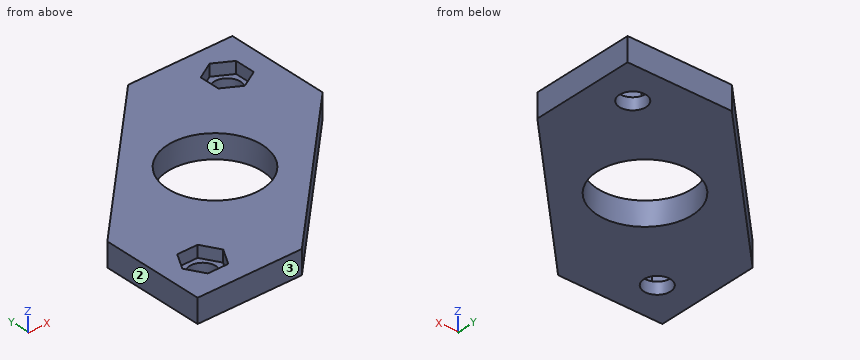
```python
from build123d import *

# Parameters (mm, degrees)
SKETCH1_R           = 8
SKETCH1_R_2         = 2.25
BOSS_EXTRUDE1_DEPTH = 4
CUT_EXTRUDE1_DEPTH  = 2


with BuildPart() as part:
    # Sketch1 → Boss-Extrude1 (new body)
    with BuildSketch(Plane.XY):
        Polygon((-4.32233047, -22), (-22, -22), (-22, -4.32233047), (4.32233047, 22), (22, 22), (22, 4.32233047), align=None)
        Circle(SKETCH1_R, mode=Mode.SUBTRACT)
        with Locations((-15.5, -15.5)):
            Circle(SKETCH1_R_2, mode=Mode.SUBTRACT)
        with Locations((15.5, 15.5)):
            Circle(SKETCH1_R_2, mode=Mode.SUBTRACT)
    extrude(amount=BOSS_EXTRUDE1_DEPTH)

    # Sketch2 → Cut-Extrude1 (cut)
    with BuildSketch(Plane.XY.offset(4)):
        Polygon((-18.964101615, -15.5), (-17.232050808, -18.5), (-13.767949192, -18.5), (-12.035898385, -15.5), (-13.767949192, -12.5), (-17.232050808, -12.5), align=None)
        Polygon((12.5, 13.767949192), (12.5, 17.232050808), (15.5, 18.964101615), (18.5, 17.232050808), (18.5, 13.767949192), (15.5, 12.035898385), align=None)
    extrude(amount=-CUT_EXTRUDE1_DEPTH, mode=Mode.SUBTRACT)


solid = part.part
```
Source: CAD feature listing. Evaluate the final solid. Frame: model axes, mm. Face numbers are marked on the shaded views. Round coordinates to 2 decimals unless told otherwise and drop trailing zeros. Write each loop counter-clockwise with the first axis right and the second up, starting at its lowest first coordinate (ties: lowest second). Pieces come first, ordered by that corner, then holes. Notation, with made-up numbers: M 56.5,7.5 L 99.5,7.5 A35 cw 99.5,44.5 Z; hole C 66.5,-10.5 d4. An arc over 180 degrees is marked long. Use CSV: the item, a comma, the result in double quotes. Start each with the question number.
Q1. First-contact query: P1, Ø1.6, axis at x = -16, z = 3.5, coming from the +Y side; P2, Ø1.6, axis at y = 15, z = 2.5, coming from the -X side; P3, Ø1.5, axis at y = -2, z = 1, coming from the +X side. Flat tips, straight axial feed; report the tip coordinate or a pass-through.
Q2. Cut plane B-B on x = -15.5. Output: boundary loops of the cut face in (y, z), plus the area to 3 significant figures.
Q3. Cut plane A-A on y = -5. Output: boundary loops of the cut face in (x, z) (3 decimals).
Q4. Line query: line 1 (Y direction, x = 0, z = 3.2); line 2 (X direction, y = -17.5, z = 0.95); line 3 (X direction, y = -15.5, z = 1.35). Output: solid intervals per line, ascending. Write a range as from..to.
Q5. Pull-direction query (Y, two-part tool) for the marked faces 1, 2 and 3; classes: +Y half, -Y half, draft (parallel to the pull), parting line (faces both ways), or undercut.
Q6. Cut plane D-D on y = 0. Output: boundary loops of the cut face in (x, z).
Q7. Cut plane C-C on z = 1.45. Output: boundary loops of the cut face in (x, y), plus the area to 3 significant figures.
Results found:
1,P1,"y = 2.48"
1,P2,"x = -3.48"
1,P3,"x = 16.43"
2,outline,"M -22,0 L -17.75,0 L -17.75,2 L -18.5,2 L -18.5,4 L -22,4 Z; M -13.25,0 L 2.18,0 L 2.18,4 L -12.5,4 L -12.5,2 L -13.25,2 Z"
2,area,"75.7 mm^2"
3,outline,"M -22,0 L -6.245,0 L -6.245,4 L -22,4 Z; M 6.245,0 L 12.678,0 L 12.678,4 L 6.245,4 Z"
4,line 1,"-17.68..-8, 8..17.68"
4,line 2,"-22..-16.53, -14.47..0.18"
4,line 3,"-22..-17.75, -13.25..2.18"
5,face 1,"undercut"
5,face 2,"draft"
5,face 3,"-Y half"
6,outline,"M -17.68,0 L -8,0 L -8,4 L -17.68,4 Z; M 8,0 L 17.68,0 L 17.68,4 L 8,4 Z"
7,outline,"M -22,-22 L -4.32,-22 L 22,4.32 L 22,22 L 4.32,22 L -22,-4.32 Z; hole C -15.5,-15.5 d4.5; hole C 0,0 d16; hole C 15.5,15.5 d4.5"
7,area,"1,010 mm^2"
